```python
from build123d import *

# Parameters (mm, degrees)
F0_W          = 174.6804863214
F0_H          = 6.394301774
F1_DEPTH      = 67.056
F2_R          = 12.7
F3_ANGLE      = 10
F4_W          = 174.6804863214
F4_H          = 3.8374643773
F4_H_2        = 3.2865575018
F4_H_3        = 4.6590082347
F4_H_4        = 3.4464076161
F4_H_5        = 3.4266933799
F4_H_6        = 3.1117796898
F5_DEPTH      = 0.635
F6_DEPTH      = 32.766
F6_DEPTH_BACK = 6.35
F7_R          = 5.08


with BuildPart() as f1:
    # F0 (on Front) → F1 (new body)
    with BuildSketch(Plane.XZ):
        with Locations((4.4365723152, 0.0675924821)):
            Rectangle(F0_W, F0_H)
    extrude(amount=F1_DEPTH)

    # F2
    f2_edges = [f1.edges().sort_by_distance(p)[0] for p in [
        (-82.903671, 0, 0.067592),
        (91.776815, 0, 0.067592),
    ]]
    fillet(f2_edges, radius=F2_R)


with BuildPart() as f1_1:
    # F3: moved
    add(f1.part.rotate(Axis((4.4365723152, 0, 3.2647433691), (1, 0, 0)), F3_ANGLE))

    # F4 (on face) → F5 (join)
    with BuildSketch(Plane(origin=(0, -0.5583039975, 3.1662993109), x_dir=(1, 0, 0), z_dir=(0, -0.1736481777, 0.984807753))):
        with Locations((4.4365723152, -18.2853909209)):
            Rectangle(F4_W, F4_H)
        with Locations((4.4365723152, -37.6678045125)):
            Rectangle(F4_W, F4_H_2)
        with Locations((4.4365723152, -27.2829253227)):
            Rectangle(F4_W, F4_H_3)
        with Locations((4.4365723152, -46.3344976306)):
            Rectangle(F4_W, F4_H_4)
        with Locations((4.4365723152, -55.3813166916)):
            Rectangle(F4_W, F4_H_5)
        with Locations((4.4365723152, -63.4787082672)):
            Rectangle(F4_W, F4_H_6)
    extrude(amount=F5_DEPTH)

    # F4 (on face) → F6 (join, two sides)
    with BuildSketch(Plane(origin=(0, -0.5583039975, 3.1662993109), x_dir=(1, 0, 0), z_dir=(0, -0.1736481777, 0.984807753))) as f6_sk:
        Polygon((-82.9036708456, -66.4382055402), (-82.9036708456, -65.0345981121), (-82.9036708456, -61.9228184223), (-82.9036708456, -57.0946633816), (-82.9036708456, -53.6679700017), (-82.9036708456, -48.0577014387), (-82.9036708456, -44.6112938225), (-82.9036708456, -39.3110832634), (-82.9036708456, -36.0245257616), (-82.9036708456, -29.61242944), (-82.9036708456, -24.9534212053), (-82.9036708456, -20.2041231096), (-82.9036708456, -16.3666587323), (-87.9721194506, -16.3666587323), (-87.9721194506, -66.4382055402), align=None)
        Polygon((91.7768154759, -61.9228184223), (91.7768154759, -65.0345981121), (91.7768154759, -66.4890832634), (96.8134328723, -66.4890832634), (96.8134328723, -16.3666587323), (91.7768154759, -16.3666587323), (91.7768154759, -20.2041231096), (91.7768154759, -24.9534212053), (91.7768154759, -29.61242944), (91.7768154759, -36.0245257616), (91.7768154759, -39.3110832634), (91.7768154759, -44.6112938225), (91.7768154759, -48.0577014387), (91.7768154759, -53.6679700017), (91.7768154759, -57.0946633816), align=None)
    extrude(amount=F6_DEPTH)
    extrude(f6_sk.sketch, amount=-F6_DEPTH_BACK)

    # F7
    f7_edges = [f1_1.edges().sort_by_distance(p)[0] for p in [
        (94.295124, -22.366073, 32.59247),
        (-85.437895, -22.366073, 32.59247),
        (-85.437895, -71.67692, 23.897637),
        (94.295124, -71.727025, 23.888802),
    ]]
    fillet(f7_edges, radius=F7_R)


solid = f1_1.part
```
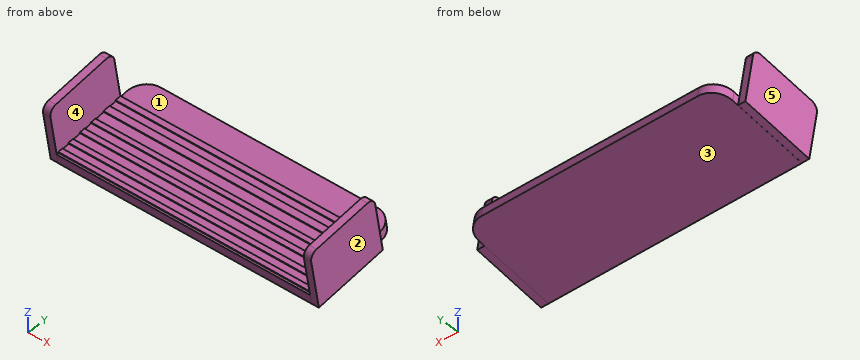
Build history of the part. All positions in model axes, mm. Face numbers are marked on the shaded views. A direction names the side the tool comes from. Round coordinates to 2 decimals unless told otherwise and drop trailing zeros. Loops run counter-clockwise (first coordinate to the right, second up) from the corner with the lowest first, then second, coordinate; pieces in that order, holes last. Notation, with made-up numbers: M 0,1 L 58,1 A18 cw 58,17 Z; hole C 25.25,-23.75 d4. An arc over 180 degrees is marked long. Answer as CSV lines item,"result".
1. Flat gauge pins, fed straight in: P1, Ø4, axis at x = 69.5, z = -7.5, coming from the -Y side; P2, Ø3, axis at x = -54, z = -2, coming from the -Y side; P3, Ø5, axis at x = -66, z = -0.5, coming from the +Y side. Where does each tip first touch, or does it go through?
Resolved:
P1,"stops at y = -66.04"
P2,"stops at y = -39.38"
P3,"stops at y = 1.1"
2. Cut at A-A on x = -34. Write the cut outline in (y, z), then the cut area to 3 significant figures.
Resolved:
outline,"M -66.04,-8.38 L -64.93,-14.68 L 1.11,-3.03 L 0,3.26 L -16.68,0.32 L -16.79,0.95 L -20.57,0.28 L -20.46,-0.34 L -25.13,-1.17 L -25.24,-0.54 L -29.83,-1.35 L -29.72,-1.98 L -36.04,-3.09 L -36.15,-2.46 L -39.38,-3.03 L -39.27,-3.66 L -44.49,-4.58 L -44.6,-3.96 L -48,-4.55 L -47.89,-5.18 L -53.41,-6.15 L -53.52,-5.53 L -56.9,-6.12 L -56.79,-6.75 L -61.54,-7.59 L -61.65,-6.96 L -64.72,-7.5 L -64.6,-8.13 Z"
area,"443 mm²"
3. 3-axis set-ups, long thin cutter, end or side, ignore diameter. For the marked faces 1 and 2: which of +Z, -Z, +X, -X, +Y, -Y reach the whole face in a straight line?
Resolved:
face 1,"+Z, +X, -X"
face 2,"+Z, -Z, +X, +Y, -Y"
4. Two-plate mould, pull along X, no slides. Class the marked faces 3, 4 and 5: released by +X, released by -X, zero draft, split by the parting line, or undercut.
Resolved:
face 3,"zero draft"
face 4,"undercut"
face 5,"released by -X"
5. Cut at C-C on z = 5. Write the cut outline in (x, y), then the cut area to 3 significant figures.
Resolved:
outline,"M -87.97,-68.34 L -82.9,-68.34 L -82.9,-17.5 L -87.97,-17.5 Z; M 91.78,-68.4 L 96.81,-68.4 L 96.81,-17.5 L 91.78,-17.5 Z"
area,"514 mm²"
6. Wall check: probe 1 along X at (y, z) = (-53, -1.5); probe 2 along Z at (x, y) = (-37, -16.5); probe 3 along Z at (x, y) = (-19, -57.5). Give the ranges that are in metal, low to high. Write a range as [from, to].
Resolved:
probe 1,"x = [-87.97, -82.9], [91.78, 96.81]"
probe 2,"z = [-6.14, 0.36]"
probe 3,"z = [-13.37, -6.87]"
7. Cut at B-B on z = 21. Write the cut outline in (x, y), then the cut area to 3 significant figures.
Resolved:
outline,"M -87.97,-70.72 L -82.9,-70.72 L -82.9,-20.32 L -87.97,-20.32 Z; M 91.78,-70.77 L 96.81,-70.77 L 96.81,-20.32 L 91.78,-20.32 Z"
area,"510 mm²"
